```python
from build123d import *

# Parameters (mm, degrees)
SKETCH2_W           = 65
SKETCH2_H           = 30
BOSS_EXTRUDE1_DEPTH = 5
SKETCH3_R           = 1.6
CUT_EXTRUDE1_DEPTH  = 37.142080737
SKETCH5_W           = 30
SKETCH5_H           = 5
BOSS_EXTRUDE2_DEPTH = 7.5
CUT_EXTRUDE2_DEPTH  = 10
SKETCH7_W           = 72.5
SKETCH7_H           = 5
BOSS_EXTRUDE3_DEPTH = 50
BOSS_EXTRUDE4_DEPTH = 5
BOSS_EXTRUDE5_DEPTH = 5
SKETCH6_R           = 1.6
CUT_EXTRUDE3_DEPTH  = 10
CUT_EXTRUDE4_DEPTH  = 79.302298817
FILLET1_R           = 2.5


with BuildPart() as part:
    # Sketch2 → Boss-Extrude1 (new body)
    with BuildSketch(Plane(origin=(0, 0, 0), x_dir=(1, 0, 0), z_dir=(0, 1, 0))):
        Rectangle(SKETCH2_W, SKETCH2_H)
    extrude(amount=BOSS_EXTRUDE1_DEPTH)

    # Sketch3 → Cut-Extrude1 (cut, through all)
    with BuildSketch(Plane(origin=(0, 5, 0), x_dir=(1, 0, 0), z_dir=(0, 1, 0))):
        with Locations(Location((-27.5, 0, 0), (0, 0, 270))):
            Circle(SKETCH3_R)
        with Locations(Location((-18, 9.5, 0), (0, 0, 270))):
            Circle(SKETCH3_R)
        with Locations(Location((-8.5, 0, 0), (0, 0, 270))):
            Circle(SKETCH3_R)
        with Locations(Location((-18, -9.5, 0), (0, 0, 270))):
            Circle(SKETCH3_R)
        with Locations(Location((18, -9.5, 0), (0, 0, 90))):
            Circle(SKETCH3_R)
        with Locations(Location((27.5, 0, 0), (0, 0, 90))):
            Circle(SKETCH3_R)
        with Locations(Location((18, 9.5, 0), (0, 0, 90))):
            Circle(SKETCH3_R)
        with Locations(Location((8.5, 0, 0), (0, 0, 90))):
            Circle(SKETCH3_R)
    extrude(amount=-CUT_EXTRUDE1_DEPTH, mode=Mode.SUBTRACT)

    # Sketch5 → Boss-Extrude2 (add)
    with BuildSketch(Plane(origin=(32.5, 0, 0), x_dir=(0, 0, -1), z_dir=(1, 0, 0))):
        with Locations((0, 2.5)):
            Rectangle(SKETCH5_W, SKETCH5_H)
    extrude(amount=BOSS_EXTRUDE2_DEPTH)

    # Sketch4 → Cut-Extrude2 (cut)
    with BuildSketch(Plane(origin=(0, 5, 0), x_dir=(1, 0, 0), z_dir=(0, 1, 0))):
        with BuildLine():
            Line((8.5, 1.6), (16, 1.6))
            ThreePointArc((16, 1.6), (17.6, 0), (16, -1.6))
            Line((16, -1.6), (8.5, -1.6))
            ThreePointArc((8.5, -1.6), (6.9, 0), (8.5, 1.6))
        make_face()
        with BuildLine():
            Line((27.5, 1.6), (35, 1.6))
            ThreePointArc((35, 1.6), (36.6, 0), (35, -1.6))
            Line((35, -1.6), (27.5, -1.6))
            ThreePointArc((27.5, -1.6), (25.9, 0), (27.5, 1.6))
        make_face()
        with BuildLine():
            Line((18, -7.9), (25.5, -7.9))
            ThreePointArc((25.5, -7.9), (27.1, -9.5), (25.5, -11.1))
            Line((25.5, -11.1), (18, -11.1))
            ThreePointArc((18, -11.1), (16.4, -9.5), (18, -7.9))
        make_face()
        with BuildLine():
            Line((18, 11.1), (25.5, 11.1))
            ThreePointArc((25.5, 11.1), (27.1, 9.5), (25.5, 7.9))
            Line((25.5, 7.9), (18, 7.9))
            ThreePointArc((18, 7.9), (16.4, 9.5), (18, 11.1))
        make_face()
    extrude(amount=-CUT_EXTRUDE2_DEPTH, mode=Mode.SUBTRACT)

    # Sketch7 → Boss-Extrude3 (add)
    with BuildSketch(Plane.XY.offset(15)):
        with Locations((3.75, 2.5)):
            Rectangle(SKETCH7_W, SKETCH7_H)
    extrude(amount=BOSS_EXTRUDE3_DEPTH)

    # Sketch10 → Boss-Extrude4 (add)
    with BuildSketch(Plane.XY.offset(25)):
        Polygon((-7.5, 5), (7.5, 5), (7.5, 22.5), (2.5, 22.5), (2.5, 17.5), (-2.5, 17.5), (-2.5, 22.5), (-7.5, 22.5), align=None)
    extrude(amount=BOSS_EXTRUDE4_DEPTH)

    # Sketch11 → Boss-Extrude5 (add)
    with BuildSketch(Plane.XY.offset(30)):
        with BuildLine():
            Line((-7.5, 22.5), (-2.5, 22.5))
            ThreePointArc((-2.5, 22.5), (0, 25), (2.5, 22.5))
            Line((2.5, 22.5), (7.5, 22.5))
            ThreePointArc((7.5, 22.5), (0, 30), (-7.5, 22.5))
        make_face()
    extrude(amount=-BOSS_EXTRUDE5_DEPTH)

    # Sketch6 → Cut-Extrude3 (cut)
    with BuildSketch(Plane.XZ):
        with Locations(Location((0, 42.5, 0), (0, 0, 270))):
            Circle(SKETCH6_R)
        with Locations(Location((0, 10, 0), (0, 0, 270))):
            Circle(SKETCH6_R)
    extrude(amount=-CUT_EXTRUDE3_DEPTH, mode=Mode.SUBTRACT)

    # Sketch14 → Cut-Extrude4 (cut, through all)
    with BuildSketch(Plane(origin=(0, 17.5, 0), x_dir=(1, 0, 0), z_dir=(0, 1, 0))):
        Polygon((-1.091089451, -25), (0, -27.5), (-1.091089451, -30), (0, -30), (1.091089451, -27.5), (0, -25), align=None)
    extrude(amount=CUT_EXTRUDE4_DEPTH, mode=Mode.SUBTRACT)

    # Fillet1
    fillet1_edges = [part.edges().sort_by_distance(p)[0] for p in [
        (-2.5, 20, 25),
        (1.767766953, 24.267766953, 25),
        (1.767766953, 24.267766953, 30),
        (-2.118693421, 23.827078817, 30),
        (-2.118693421, 23.827078817, 25),
        (2.5, 20, 25),
        (0, 17.5, 25),
        (2.5, 20, 30),
        (0, 17.5, 30),
        (-2.5, 20, 30),
    ]]
    fillet(fillet1_edges, radius=FILLET1_R - 0.0001)  # a hair under: the kernel refuses the full size


solid = part.part
```
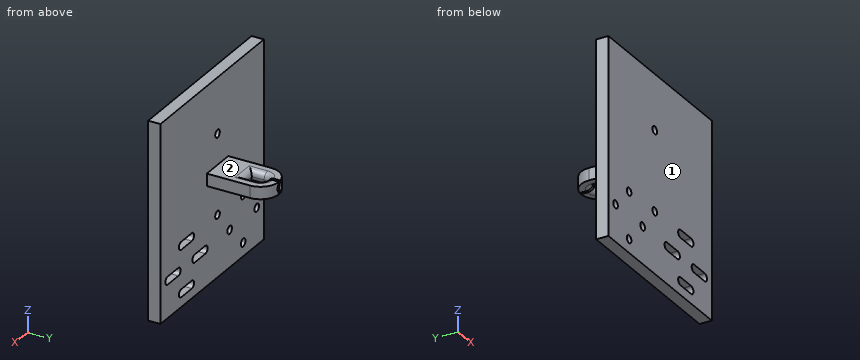
Model file for the job. Use its own axes, mm. Face numbers are marked on the shaded views. A direction names the side the tool comes from. Coordinates: 2 decimals unless noted, no trailing zeros. Write each loop counter-clockwise with the first axis right and the second up, starting at its lowest first coordinate (ties: lowest second). Pieces come first, ordered by that corner, then holes. Notation, with made-up numbers: (32.25, 51) - (72.25, 51) arc R15 cw to (72.25, 76) - close; hole circle Ø9 at (83, -7). An arc over 180 degrees is marked (long way). One line per item, written item: value. Start each with the question number.
1. Slice it at A-A (x = -18). Write the cut outline in (y, z), plus the area to 3 significant figures.
2. Slice it at D-D (x = -8.5). Write the cut outline in (y, z), plus the area to 3 significant figures.
3. Slice it at C-C (z = -9.5). Write the cut outline in (x, y).
4. Flat gauge pins, fed straight in: pin 1 (2.5 mm diameter, centred on y = 16.5, z = 28, fed in from +X); pin 2 (4 mm diameter, centred on x = 0, z = 10, fed in from +Y); pin 3 (6 mm diameter, centred on x = -6.5, z = 29.5, fed in from +Y). Where does each tip first touch, or does it go through?
5. Tool access for the marked faces 1 and 2: list every direction of +Z, -Z, +X, -X, +Y, -Y with a clear straight run to the whole face (end or side of a thin tool).
6. Probe line 1 (X direction, y = 1, z = 0); line 2 (X direction, y = 1, z = 9); line 3 (X direction, y = 3.05, z = 10). List the from-to ranges inside material, lowest first. Write a range as from..to.
Answers below:
1. outline: (0, -15) - (5, -15) - (5, -11.1) - (0, -11.1) - close; (0, -7.9) - (5, -7.9) - (5, 7.9) - (0, 7.9) - close; (0, 11.1) - (5, 11.1) - (5, 65) - (0, 65) - close
1. area: 368 mm^2
2. outline: (0, -15) - (5, -15) - (5, -1.6) - (0, -1.6) - close; (0, 1.6) - (5, 1.6) - (5, 65) - (0, 65) - close
2. area: 384 mm^2
3. outline: (-32.5, 0) - (-19.6, 0) - (-19.6, 5) - (-32.5, 5) - close; (-16.4, 0) - (16.4, 0) - (16.4, 5) - (-16.4, 5) - close; (27.1, 0) - (40, 0) - (40, 5) - (27.1, 5) - close
4. pin 1: stops at x = 7.5
4. pin 2: stops at y = 5
4. pin 3: stops at y = 29.13
5. face 1: +Z, -Z, +X, -X, -Y
5. face 2: +Z, +X, -X, +Y
6. line 1: x = -32.5..-29.1, -25.9..-10.1, -6.9..6.9, 17.6..25.9, 36.6..40
6. line 2: x = -32.5..-19.52, -16.48..-1.25, 1.25..16.48, 27.02..40
6. line 3: x = -32.5..-19.52, -16.48..-1.6, 1.6..16.48, 27.02..40
